Source: CAD feature listing. Evaluate the final solid. Frame: model axes, mm. A direction names the side the tool comes from. Coordinates: 2 decimals unless noted, no trailing zeros. Order: outer loops, then holes, each group sorted by start corner. A loop starts at its lowest first (then second) coordinate and runs counter-clockwise, first axis right, second up. Notation, with made-up numbers: (32, 48) -> (39, 48) arc R20 cw to (39, 81) -> close; hole circle Ø6 at (30.25, 55.25). An arc over 180 degrees is marked (long way). Write item = value, one per line. Start each with the question number.
Item 1: Section query C-C (z = -8). Output: boundary loops of the cut face in (x, y), then the cut area to 3 significant figures.
Item 2: Contact query for flat-ended pins moving along their axis: pin 1 (4.5 mm diameter, centred on y = 10, z = -9, fed in from +X); pin 2 (4 mm diameter, centred on x = 0, z = -5, fed in from +Y); pin 3 (1.5 mm diameter, centred on x = -9, z = -9, fed in from +Y); pin 4 (4 mm diameter, centred on x = 1, z = -7, fed in from +Y). Output: stop coordinate, or through.
Item 3: Ray query, line 1 along Z through (x, y) = (0, 5.5); line 2 along Y through (x, z) = (5, -13.25); line 3 along Y through (x, z) = (-7.5, -10). Return the intervals inside material, ascending. Write a range as [from, to].
Item 4: Mould query, pull axis Y, two halves, no side actions, for faces 4 (the flat face through (-8, 5, -15)), 5 (the flat face through (0, 14, -15)), 6 (the flat face through (0, 18, 0)). Classes: released by +Y, released by -Y, zero draft, split by the parting line, or undercut.
Item 5: Section query D-D (y = 6.5). Output: boundary loops of the cut face in (x, z), then the cut area to 3 significant figures.
Item 6: Section query B-B (x = 0). Output: boundary loops of the cut face in (y, z).
Item 7: Section query A-A (z = -5). Output: boundary loops of the cut face in (x, y), then the cut area to 3 significant figures.
Item 8: Set-up query: faces 1 (the flat face through (9, 5, -15)), 2 (the flat face through (-7, 13, -18)), 3 (the flat face through (0, 16, -9)). Return all of +Z, -Z, +X, -X, +Y, -Y with unobstructed straight access to the full face (end or side cutting, diameter ignored); none if empty.
```python
from build123d import *

# Parameters (mm, degrees)
F0_W     = 14
F0_H     = 4
F0_H_2   = 5
F1_DEPTH = 30
F2_W     = 14
F2_H     = 5
F3_DEPTH = 15
F4_R     = 2.5
F5_DEPTH = 25


with BuildPart() as f1:
    # F0 (on Top) → F1 (new body)
    with BuildSketch(Plane.XY):
        with Locations((0, 18)):
            Rectangle(F0_W, F0_H)
        with Locations((0, 13.5)):
            Rectangle(F0_W, F0_H_2)
        Polygon((-10, 5), (-10, 0), (10, 0), (10, 5), (7, 5), (7, 11), (-7, 11), (-7, 5), align=None)
    extrude(amount=-F1_DEPTH)

    # F2 (on face) → F3 (cut)
    with BuildSketch(Plane.XY):
        with Locations((0, 13.5)):
            Rectangle(F2_W, F2_H)
    extrude(amount=-F3_DEPTH, mode=Mode.SUBTRACT)

    # F4 (on face) → F5 (cut)
    with BuildSketch(Plane(origin=(0, 20, 0), x_dir=(-1, 0, 0), z_dir=(0, 1, 0))):
        with Locations((0, -5)):
            Circle(F4_R)
    extrude(amount=-F5_DEPTH, mode=Mode.SUBTRACT)


solid = f1.part
```
Computed:
q1.outline = (-10, 0) -> (10, 0) -> (10, 5) -> (7, 5) -> (7, 11) -> (-7, 11) -> (-7, 5) -> (-10, 5) -> close; (-7, 16) -> (7, 16) -> (7, 20) -> (-7, 20) -> close
q1.area = 240 mm^2
q2.pin_1 = 7
q2.pin_2 = through
q2.pin_3 = 5
q2.pin_4 = 20
q3.line_1 = [-30, -7.5], [-2.5, 0]
q3.line_2 = [0, 11], [16, 20]
q3.line_3 = [0, 5]
q4.face_4 = released by +Y
q4.face_5 = undercut
q4.face_6 = zero draft
q5.outline = (-7, -30) -> (7, -30) -> (7, 0) -> (-7, 0) -> close; hole circle Ø5 at (0, -5)
q5.area = 400 mm^2
q6.outline = (0, -30) -> (20, -30) -> (20, -7.5) -> (16, -7.5) -> (16, -15) -> (11, -15) -> (11, -7.5) -> (0, -7.5) -> close; (0, -2.5) -> (11, -2.5) -> (11, 0) -> (0, 0) -> close; (16, -2.5) -> (20, -2.5) -> (20, 0) -> (16, 0) -> close
q7.outline = (-10, 0) -> (-2.5, 0) -> (-2.5, 11) -> (-7, 11) -> (-7, 5) -> (-10, 5) -> close; (-7, 16) -> (-2.5, 16) -> (-2.5, 20) -> (-7, 20) -> close; (2.5, 0) -> (10, 0) -> (10, 5) -> (7, 5) -> (7, 11) -> (2.5, 11) -> close; (2.5, 16) -> (7, 16) -> (7, 20) -> (2.5, 20) -> close
q7.area = 165 mm^2
q8.face_1 = +Z, -Z, +X, +Y
q8.face_2 = +Z, -Z, -X, +Y
q8.face_3 = +Z, +X, -X
